```python
from build123d import *

# Parameters (mm, degrees)
SKETCH_1_R          = 2.1
EXTRUDE_1_DEPTH     = 3
FILLET_1_R          = 5
CUT_EXTRUDE_1_DEPTH = 127.052568399


with BuildPart() as part:
    # 草图1 → 凸台-拉伸1 (new body)
    with BuildSketch(Plane(origin=(0, 0, 0), x_dir=(1, 0, 0), z_dir=(0, 1, 0))):
        with BuildLine():
            Line((-5, 37), (30, 37))
            Line((30, 37), (47.5, -5))
            Line((47.5, -5), (42, -5))
            ThreePointArc((42, -5), (41, -4), (40, -5))
            Line((40, -5), (40, -10))
            ThreePointArc((40, -10), (41, -11), (42, -10))
            Line((42, -10), (119.5, -10))
            Line((119.5, -10), (119.5, -40))
            Line((119.5, -40), (-94.5, -40))
            Line((-94.5, -40), (-94.5, -10))
            Line((-94.5, -10), (-17, -10))
            ThreePointArc((-17, -10), (-16, -11), (-15, -10))
            Line((-15, -10), (-15, -5))
            ThreePointArc((-15, -5), (-16, -4), (-17, -5))
            Line((-17, -5), (-22.5, -5))
            Line((-22.5, -5), (-5, 37))
        make_face()
        with Locations(Location((0, 30, 0), (0, 0, 270))):
            Circle(SKETCH_1_R, mode=Mode.SUBTRACT)
        with Locations(Location((0, 0, 0), (0, 0, 270))):
            Circle(SKETCH_1_R, mode=Mode.SUBTRACT)
        with Locations(Location((-89.5, -15, 0), (0, 0, 270))):
            Circle(SKETCH_1_R, mode=Mode.SUBTRACT)
        with Locations(Location((-39.5, -15, 0), (0, 0, 270))):
            Circle(SKETCH_1_R, mode=Mode.SUBTRACT)
        with Locations(Location((-89.5, -35, 0), (0, 0, 270))):
            Circle(SKETCH_1_R, mode=Mode.SUBTRACT)
        with Locations(Location((-39.5, -35, 0), (0, 0, 270))):
            Circle(SKETCH_1_R, mode=Mode.SUBTRACT)
        with Locations(Location((64.5, -35, 0), (0, 0, 90))):
            Circle(SKETCH_1_R, mode=Mode.SUBTRACT)
        with Locations(Location((114.5, -35, 0), (0, 0, 90))):
            Circle(SKETCH_1_R, mode=Mode.SUBTRACT)
        with Locations(Location((64.5, -15, 0), (0, 0, 90))):
            Circle(SKETCH_1_R, mode=Mode.SUBTRACT)
        with Locations(Location((114.5, -15, 0), (0, 0, 90))):
            Circle(SKETCH_1_R, mode=Mode.SUBTRACT)
        with Locations(Location((25, 0, 0), (0, 0, 90))):
            Circle(SKETCH_1_R, mode=Mode.SUBTRACT)
        with Locations(Location((25, 30, 0), (0, 0, 90))):
            Circle(SKETCH_1_R, mode=Mode.SUBTRACT)
        with BuildLine():
            Line((2, -10), (23, -10))
            ThreePointArc((23, -10), (24, -11), (25, -10))
            Line((25, -10), (25, -5))
            ThreePointArc((25, -5), (24, -4), (23, -5))
            Line((23, -5), (2, -5))
            ThreePointArc((2, -5), (1, -4), (0, -5))
            Line((0, -5), (0, -10))
            ThreePointArc((0, -10), (1, -11), (2, -10))
        make_face(mode=Mode.SUBTRACT)
    extrude(amount=EXTRUDE_1_DEPTH)

    # 圆角1
    fillet_1_edges = [part.edges().sort_by_distance(p)[0] for p in [
        (-5, 1.5, -37),
        (30, 1.5, -37),
        (119.5, 1.5, 10),
        (119.5, 1.5, 40),
        (-94.5, 1.5, 40),
        (-94.5, 1.5, 10),
    ]]
    fillet(fillet_1_edges, radius=FILLET_1_R)

    # 草图2 → 切除-拉伸1 (cut, through all)
    with BuildSketch(Plane(origin=(0, 3, 0), x_dir=(1, 0, 0), z_dir=(0, 1, 0))):
        with BuildLine():
            Line((-89.5, -29.083920217), (-89.5, -19.708131846))
            ThreePointArc((-89.5, -19.708131846), (-89.060628809, -18.880064615), (-88.128609324, -18.779655155))
            Line((-88.128609324, -18.779655155), (-52.398938938, -33.071523309))
            ThreePointArc((-52.398938938, -33.071523309), (-51.788373228, -34.189107521), (-52.770329614, -35))
            Line((-52.770329614, -35), (-83.583920217, -35))
            ThreePointArc((-83.583920217, -35), (-84.229417441, -34.763762616), (-84.569933514, -34.166666667))
            ThreePointArc((-84.569933514, -34.166666667), (-85.964466094, -31.464466094), (-88.666666667, -30.069933514))
            ThreePointArc((-88.666666667, -30.069933514), (-89.263762616, -29.729417441), (-89.5, -29.083920217))
        make_face()
        with BuildLine():
            Line((-45.416079783, -15), (-76.229670386, -15))
            ThreePointArc((-76.229670386, -15), (-77.211626772, -15.810892479), (-76.601061062, -16.928476691))
            Line((-76.601061062, -16.928476691), (-40.871390676, -31.220344845))
            ThreePointArc((-40.871390676, -31.220344845), (-39.939371191, -31.119935385), (-39.5, -30.291868154))
            Line((-39.5, -30.291868154), (-39.5, -20.916079783))
            ThreePointArc((-39.5, -20.916079783), (-39.736237384, -20.270582559), (-40.333333333, -19.930066486))
            ThreePointArc((-40.333333333, -19.930066486), (-43.035533906, -18.535533906), (-44.430066486, -15.833333333))
            ThreePointArc((-44.430066486, -15.833333333), (-44.770582559, -15.236237384), (-45.416079783, -15))
        make_face()
        with BuildLine():
            Line((64.5, -30.291868154), (64.5, -20.916079783))
            ThreePointArc((64.5, -20.916079783), (64.736237384, -20.270582559), (65.333333333, -19.930066486))
            ThreePointArc((65.333333333, -19.930066486), (68.035533906, -18.535533906), (69.430066486, -15.833333333))
            ThreePointArc((69.430066486, -15.833333333), (69.770582559, -15.236237384), (70.416079783, -15))
            Line((70.416079783, -15), (101.229670386, -15))
            ThreePointArc((101.229670386, -15), (102.211626772, -15.810892479), (101.601061062, -16.928476691))
            Line((101.601061062, -16.928476691), (65.871390676, -31.220344845))
            ThreePointArc((65.871390676, -31.220344845), (64.939371191, -31.119935385), (64.5, -30.291868154))
        make_face()
        with BuildLine():
            Line((77.770329614, -35), (108.583920217, -35))
            ThreePointArc((108.583920217, -35), (109.229417441, -34.763762616), (109.569933514, -34.166666667))
            ThreePointArc((109.569933514, -34.166666667), (110.964466094, -31.464466094), (113.666666667, -30.069933514))
            ThreePointArc((113.666666667, -30.069933514), (114.263762616, -29.729417441), (114.5, -29.083920217))
            Line((114.5, -29.083920217), (114.5, -19.708131846))
            ThreePointArc((114.5, -19.708131846), (114.060628809, -18.880064615), (113.128609324, -18.779655155))
            Line((113.128609324, -18.779655155), (77.398938938, -33.071523309))
            ThreePointArc((77.398938938, -33.071523309), (76.788373228, -34.189107521), (77.770329614, -35))
        make_face()
        with BuildLine():
            Line((-14.583333333, 0), (-7.505553499, 0))
            ThreePointArc((-7.505553499, 0), (-7.005553499, 0.133974596), (-6.639528096, 0.5))
            Line((-6.639528096, 0.5), (-5.133974596, 3.107695155))
            ThreePointArc((-5.133974596, 3.107695155), (-5.034074174, 3.348876109), (-5, 3.607695155))
            Line((-5, 3.607695155), (-5, 21.6))
            ThreePointArc((-5, 21.6), (-5.803883865, 22.580580676), (-6.923076923, 21.984615385))
            Line((-6.923076923, 21.984615385), (-15.506410256, 1.384615385))
            ThreePointArc((-15.506410256, 1.384615385), (-15.415383628, 0.445299804), (-14.583333333, 0))
        make_face()
        with BuildLine():
            Line((30, 3.607695155), (30, 21.6))
            ThreePointArc((30, 21.6), (30.803883865, 22.580580676), (31.923076923, 21.984615385))
            Line((31.923076923, 21.984615385), (40.506410256, 1.384615385))
            ThreePointArc((40.506410256, 1.384615385), (40.415383628, 0.445299804), (39.583333333, 0))
            Line((39.583333333, 0), (32.505553499, 0))
            ThreePointArc((32.505553499, 0), (32.005553499, 0.133974596), (31.639528096, 0.5))
            Line((31.639528096, 0.5), (30.133974596, 3.107695155))
            ThreePointArc((30.133974596, 3.107695155), (30.034074174, 3.348876109), (30, 3.607695155))
        make_face()
        with BuildLine():
            Line((3, 23.07179677), (3, 6.92820323))
            ThreePointArc((3, 6.92820323), (3.133974596, 6.42820323), (3.5, 6.062177826))
            ThreePointArc((3.5, 6.062177826), (5.281992573, 4.593533984), (6.489173676, 2.625))
            ThreePointArc((6.489173676, 2.625), (6.857181493, 2.170843802), (7.416198487, 2))
            Line((7.416198487, 2), (17.583801513, 2))
            ThreePointArc((17.583801513, 2), (18.142818507, 2.170843802), (18.510826324, 2.625))
            ThreePointArc((18.510826324, 2.625), (19.718007427, 4.593533984), (21.5, 6.062177826))
            ThreePointArc((21.5, 6.062177826), (21.866025404, 6.42820323), (22, 6.92820323))
            Line((22, 6.92820323), (22, 23.07179677))
            ThreePointArc((22, 23.07179677), (21.866025404, 23.57179677), (21.5, 23.937822174))
            ThreePointArc((21.5, 23.937822174), (19.168900851, 26.127238361), (18.054902808, 29.125))
            ThreePointArc((18.054902808, 29.125), (17.724183895, 29.75), (17.062746067, 30))
            Line((17.062746067, 30), (7.937253933, 30))
            ThreePointArc((7.937253933, 30), (7.275816105, 29.75), (6.945097192, 29.125))
            ThreePointArc((6.945097192, 29.125), (5.831099149, 26.127238361), (3.5, 23.937822174))
            ThreePointArc((3.5, 23.937822174), (3.133974596, 23.57179677), (3, 23.07179677))
        make_face()
        with BuildLine():
            Line((1.911922611, -16.928476691), (23.088077389, -16.928476691))
            ThreePointArc((23.088077389, -16.928476691), (23.974191323, -17.465009221), (23.909447355, -18.4988725))
            Line((23.909447355, -18.4988725), (13.321369966, -33.74570394))
            ThreePointArc((13.321369966, -33.74570394), (12.5, -34.175308131), (11.678630034, -33.74570394))
            Line((11.678630034, -33.74570394), (1.090552645, -18.4988725))
            ThreePointArc((1.090552645, -18.4988725), (1.025808677, -17.465009221), (1.911922611, -16.928476691))
        make_face()
        with BuildLine():
            Line((-32.5, -17.928476691), (-32.5, -27.485287367))
            ThreePointArc((-32.5, -27.485287367), (-31.957581581, -28.37445501), (-30.918761806, -28.299020838))
            Line((-30.918761806, -28.299020838), (-17.53922686, -18.742210162))
            ThreePointArc((-17.53922686, -18.742210162), (-17.168169545, -17.62329926), (-18.120465053, -16.928476691))
            Line((-18.120465053, -16.928476691), (-31.5, -16.928476691))
            ThreePointArc((-31.5, -16.928476691), (-32.207106781, -17.22136991), (-32.5, -17.928476691))
        make_face()
        with BuildLine():
            Line((-23.997185346, -33.186266529), (-4.489724414, -19.252365863))
            ThreePointArc((-4.489724414, -19.252365863), (-3.737550205, -19.080817203), (-3.087116254, -19.495703525))
            Line((-3.087116254, -19.495703525), (6.589203652, -33.429604191))
            ThreePointArc((6.589203652, -33.429604191), (6.653947621, -34.463467469), (5.767833687, -35))
            Line((5.767833687, -35), (-23.415947152, -35))
            ThreePointArc((-23.415947152, -35), (-24.368242661, -34.305177431), (-23.997185346, -33.186266529))
        make_face()
        with BuildLine():
            Line((28.087116254, -19.495703525), (18.410796348, -33.429604191))
            ThreePointArc((18.410796348, -33.429604191), (18.346052379, -34.463467469), (19.232166313, -35))
            Line((19.232166313, -35), (48.415947152, -35))
            ThreePointArc((48.415947152, -35), (49.368242661, -34.305177431), (48.997185346, -33.186266529))
            Line((48.997185346, -33.186266529), (29.489724414, -19.252365863))
            ThreePointArc((29.489724414, -19.252365863), (28.737550205, -19.080817203), (28.087116254, -19.495703525))
        make_face()
        with BuildLine():
            Line((55.918761806, -28.299020838), (42.53922686, -18.742210162))
            ThreePointArc((42.53922686, -18.742210162), (42.168169545, -17.62329926), (43.120465053, -16.928476691))
            Line((43.120465053, -16.928476691), (56.5, -16.928476691))
            ThreePointArc((56.5, -16.928476691), (57.207106781, -17.22136991), (57.5, -17.928476691))
            Line((57.5, -17.928476691), (57.5, -27.485287367))
            ThreePointArc((57.5, -27.485287367), (56.957581581, -28.37445501), (55.918761806, -28.299020838))
        make_face()
    extrude(amount=-CUT_EXTRUDE_1_DEPTH, mode=Mode.SUBTRACT)


solid = part.part
```
Model file for the job. Use its own axes, mm. Coordinates: 2 decimals unless noted, no trailing zeros. Write each loop counter-clockwise with the first axis right and the second up, starting at its lowest first coordinate (ties: lowest second). Pieces come first, ordered by that corner, then holes. Notation, with made-up numbers: (-29, 80) - (28, 80) arc R25 cw to (28, 108) - close; hole circle Ø1 at (36, 0). An arc over 180 degrees is marked (long way). One line per item, written item: value. Start each with the question number.
1. Mould opens along Z. For faces 1 (the cylindrical face through (0.631, 1.479, 2.003)), 2 (the cylindrical face through (-93.07, 1.52, 38.5)), 3 (the flat face through (13, 3, 16)), 4 (the cylindrical face through (23.23, 1.48, -1.13)) say: released by +Z, released by -Z, zero draft, split by the parting line, or undercut.
2. Slice it at A-A (x = 53). Write the cut outline in (y, z), plus the area to 3 significant figures.
3. Flat gauge pins, fed straight in: pin 1 (6.5 mm diameter, centred on x = 25, z = -30, fed in from -Y); pin 2 (1.5 mm diameter, centred on y = 1.5, z = 7, fed in from -X); pin 3 (3.5 mm diameter, centred on x = 114.5, z = 15, fed in from -Y); pin 4 (0.9 mm diameter, centred on x = -50, y = 1.5, fed in from -Z). Where does each tip first touch, or does it go through?
4. Probe line 1 (Z direction, x = -11, y = 0.55); line 2 (Z direction, x = -12, y = 1.65); line 3 (X direction, y = 1.5, z = 1). List the from-to ranges inside material, lowest first. Write a range as from..to.
5. Slice it at C-C (z = -10). Write the cut outline in (x, y), plus the area to 3 significant figures.
6. Slice it at B-B (x = -12.5). Write the cut outline in (y, z).
7. Slice it at D-D (x = 95). Write the cut outline in (y, z), plus the area to 3 significant figures.
Answers below:
1. face 1: undercut
1. face 2: released by +Z
1. face 3: zero draft
1. face 4: undercut
2. outline: (0, 10) - (3, 10) - (3, 16.93) - (0, 16.93) - close; (0, 26.21) - (3, 26.21) - (3, 40) - (0, 40) - close
2. area: 62.1 mm^2
3. pin 1: stops at y = 0
3. pin 2: stops at x = -15
3. pin 3: passes through
3. pin 4: stops at z = 10
4. line 1: z = -22.6..-12.2, 0..23.9, 35..40
4. line 2: z = -20.2..-9.8, 0..24.62, 35..40
4. line 3: x = -20.83..-1.85, 1.85..23.15, 26.85..45.83
5. outline: (-16.25, 0) - (-11.92, 0) - (-11.92, 3) - (-16.25, 3) - close; (-5, 0) - (3, 0) - (3, 3) - (-5, 3) - close; (22, 0) - (30, 0) - (30, 3) - (22, 3) - close; (36.92, 0) - (41.25, 0) - (41.25, 3) - (36.92, 3) - close
5. area: 74.0 mm^2
6. outline: (0, -19) - (3, -19) - (3, -8.6) - (0, -8.6) - close; (0, 0) - (3, 0) - (3, 24.97) - (0, 24.97) - close; (0, 35) - (3, 35) - (3, 40) - (0, 40) - close
7. outline: (0, 10) - (3, 10) - (3, 15) - (0, 15) - close; (0, 19.57) - (3, 19.57) - (3, 26.03) - (0, 26.03) - close; (0, 35) - (3, 35) - (3, 40) - (0, 40) - close
7. area: 49.4 mm^2
